Geometry check sheet. Reference: the model listing, model coordinates, mm. A direction names the side the tool comes from. Round coordinates to 2 decimals unless told otherwise and drop trailing zeros. Order: outer loops, then holes, each group sorted by start corner. A loop starts at its lowest first (then second) coordinate and runs counter-clockwise, first axis right, second up. Notation, with made-up numbers: (-37, -32) - (7, -32) arc R10 cw to (7, -13) - close; hole circle Ø6 at (7.25, -1). An arc over 180 degrees is marked (long way). Use a Markdown table: item, result. Add a question column.
(1) Section check B-B on y = 43. Record the boundary of the cut face in (x, z).
(2) Section check A-A on y = 27.5. Record the boundary of the cut face in (x, z) (3 decimals), then the cut area to 3 significant figures.
(3) Mould release check, pull along X, two halves, no side actions. Record for faces 1 (the face through (23.74, 42.598, 26.956)), 2 (the face through (-12.125, 27, -41)), 3 (the face through (5, 45.803, 36)), 4 (the face through (-52, 27, 0.375)): released by +X, released by -X, zero draft, split by the parting line, or undercut.
(4) Section check C-C on y = 11.5. Record the boundary of the cut face in (x, z), then the cut area to 3 significant figures.
(5) Gauge pin test, flat ends, axial feed: P1, Ø1, axis at x = -5.5, z = -30.5, coming from the -Y side; P2, Ø6, axis at y = 23.5, z = -32, coming from the -X side; P3, Ø0.8, axis at y = 29, z = 41, coming from the -X side. Record the tip position at first contact, or that the pin passes through.
(6) Thickness scan on line 1 along Y through (x, z) = (-33.5, 0.5); line 2 along X through (y, z) = (12, -27.5); line 3 along X through (y, z) = (40.5, -4.5). Record the ranges inside material, lowest first. Write a range as [from, to].
(7) Access from +Z, -Z, +X, -X, +Y, -Y to the whole of each face (thin tool, end or side, straight path). Record for faces 5 (the face through (-10.706, 27, 41)), 6 (the face through (2.07, 42.6, -12.37)), 7 (the face through (-6.98, 49.86, -33.81)).
```python
from build123d import *

# Parameters (mm, degrees)
ESQUISSE1_W        = 15.8
ESQUISSE1_H        = 6.5
ESQUISSE1_W_2      = 5.2
ESQUISSE1_H_2      = 8
ESQUISSE2_W        = 2
ESQUISSE2_H        = 2.5
BOSS_EXTRU_2_DEPTH = 25
ESQUISSE3_W        = 2.5
ESQUISSE3_H        = 2
ESQUISSE3_W_2      = 2
ESQUISSE3_H_2      = 2.5
BOSS_EXTRU_3_DEPTH = 25


with BuildPart() as part:
    # Esquisse1 → Révolution1 (revolve)
    with BuildSketch(Plane.XY, mode=Mode.PRIVATE) as r_volution1_sk:
        Polygon((32.884729147, 39.302631579), (29.884729147, 39.302631579), (33.372699072, -6.697368421), (36.084729147, -6.697368421), align=None)
        Polygon((27.884729147, 45.802631579), (22.684729147, 45.802631579), (22.684729147, 39.302631579), (29.884729147, 39.302631579), (32.884729147, 39.302631579), (32.884729147, 45.802631579), align=None)
        with Locations((14.784729147, 42.552631579)):
            Rectangle(ESQUISSE1_W, ESQUISSE1_H)
        with Locations((25.284729147, 49.802631579)):
            Rectangle(ESQUISSE1_W_2, ESQUISSE1_H_2)
    revolve(r_volution1_sk.sketch.rotate(Axis((-11.415270853, 52.302631579, 0), (0, -1, 0)), 180), axis=Axis((-11.415270853, 52.302631579, 0), (0, -1, 0)))

    # Esquisse2 → Boss.-Extru.2 (add)
    with BuildSketch(Plane.XZ.offset(-39.302631579)):
        with Locations((-11.124553999, -41.298976788)):
            Rectangle(ESQUISSE2_W, ESQUISSE2_H)
    extrude(amount=BOSS_EXTRU_2_DEPTH)

    # Esquisse3 → Boss.-Extru.3 (add)
    with BuildSketch(Plane.XZ.offset(-39.302631579)):
        with Locations((-52.710541461, -0.6250003)):
            Rectangle(ESQUISSE3_W, ESQUISSE3_H)
        with Locations((-11.706072968, 41.298976187)):
            Rectangle(ESQUISSE3_W_2, ESQUISSE3_H_2)
    extrude(amount=BOSS_EXTRU_3_DEPTH)


solid = part.part
```
Check sheet entries:
| question | item | result |
|---|---|---|
| 1 | outline | circle Ø88.6 at (-11.42, 0); hole circle Ø36.6 at (-11.42, 0) |
| 2 | outline | circle Ø90.242 at (-11.415, 0); hole (-53.609, 0.375) - (-51.461, 0.375) - (-51.461, -1.625) - (-53.579, -1.625) arc R42.195 ccw to (-12.125, -42.189) - (-12.125, -40.049) - (-10.125, -40.049) - (-10.125, -42.175) arc R42.195 ccw to (-10.706, 42.189) - (-10.706, 40.049) - (-12.706, 40.049) - (-12.706, 42.175) arc R42.195 ccw to start |
| 2 | area | 816 mm2 |
| 3 | face 1 | split by the parting line |
| 3 | face 2 | undercut |
| 3 | face 3 | zero draft |
| 3 | face 4 | undercut |
| 4 | outline | circle Ø92.47 at (-11.42, 0); hole circle Ø86.82 at (-11.42, 0) |
| 4 | area | 796 mm2 |
| 5 | P1 | stops at y = 39.3 |
| 5 | P2 | stops at x = -46.36 |
| 5 | P3 | stops at x = -30.86 |
| 6 | line 1 | y = [39.3, 45.8] |
| 6 | line 2 | x = [-48.54, -44.95], [22.12, 25.71] |
| 6 | line 3 | x = [-55.49, -29.15], [6.32, 32.66] |
| 7 | face 5 | -Y |
| 7 | face 6 | +Y, -Y |
| 7 | face 7 | +Y |
